Source: CAD feature listing. Evaluate the final solid. Frame: model axes, mm. A direction names the side the tool comes from. Round coordinates to 2 decimals unless told otherwise and drop trailing zeros. Order: outer loops, then holes, each group sorted by start corner. A loop starts at its lowest first (then second) coordinate and runs counter-clockwise, first axis right, second up. Notation, with made-up numbers: M 5.5,22 L 42.5,22 A29 cw 42.5,52 Z; hole C 66.5,-1.5 d8. An arc over 180 degrees is marked long. Answer in a Markdown table with one row per item. Add a question column.
```python
from build123d import *

# Parameters (mm, degrees)
F1_DEPTH = 2.0574
F2_R     = 2.54


with BuildPart() as f1:
    # F0 (on Top) → F1 (new body)
    with BuildSketch(Plane.XY):
        Polygon((-19.05, -6.831449), (0, -7.122084), (0, -4.836785), (-19.05, -4.546149), (-19.05, 5.615033), (-21.59, 5.653784), (-21.59, -16.95388), (-19.05, -16.992631), align=None)
        with BuildLine():
            Line((0, -7.122084), (3.032153, -7.168344))
            ThreePointArc((3.032153, -7.168344), (7.041994, 3.104817), (-2.545553, -2.344551))
            Line((-2.545553, -2.344551), (-0.515844, -2.007228))
            ThreePointArc((-0.515844, -2.007228), (5.158216, 1.472099), (3.187775, -4.885419))
            Line((3.187775, -4.885419), (0, -4.836785))
            Line((0, -4.836785), (0, -7.122084))
        make_face()
    extrude(amount=F1_DEPTH)

    # F2
    f2_edges = [f1.edges().sort_by_distance(p)[0] for p in [
        (-19.05, -6.831449, 1.0287),
        (-19.05, -4.546149, 1.0287),
    ]]
    fillet(f2_edges, radius=F2_R)


solid = f1.part
```
(1) Cut plane A-A (z = 0.6). Return loops of the section in (x, y), and give its area (3 significant figures).
(2) Cut plane B-B (y = -0.25). Return loops of the section in (x, z).
(3) Line query: line 1 (X direction, y = -0.75, z = 1.6); line 2 (X direction, y = 1.25, z = 1.55); line 3 (Y direction, x = 1, z = 0.95). Output: solid intervals per line, ascending. Write a range as from..to.
(4) Access query for faces 1 (the face through (-18.27, -7.58, 1.04)), 2 (the face through (7.19, 2.97, 1.01)), 3 (the face through (-18.3, -3.847, 1.043)). Directions: +Z, -Z, +X, -X, +Y, -Y. A direction counts if a zero-diameter tool reaches every point of the face in a straight line with its end or side. Return the directions, or none.
(5) Cut plane D-D (y = 2.75). Return loops of the section in (x, z).
(6) Pin query (flat end, axial travel): pin 1 (1 mm diameter, centred on y = -9.5, z = 0.5, fed in from +X); pin 2 (1.5 mm diameter, centred on x = -14.5, y = -4.5, fed in from -Z); pin 3 (0.6 mm diameter, centred on y = -13, z = 1.5, fed in from +X). Return the tip coordinate at first contact, or that it passes through.
(7) Cut plane C-C (x = 2.5). Return loops of the section in (y, z).
(8) Draft query along X for faces 4 (the face through (-19.05, -13, 1)), 5 (the face through (-9, -5, 2.057)), 6 (the face through (-1.545, -2.178, 1.014)). Return one class per face: +X half, -X half, draft (parallel to the pull), parting line (faces both ways), or undercut.
Answer list:
| question | item | result |
|---|---|---|
| 1 | outline | M -21.59,-16.95 L -19.05,-16.99 L -19.05,-9.41 A2.54 cw -16.47,-6.87 L 3.03,-7.17 A5.85 ccw long -2.55,-2.34 L -0.52,-2.01 A3.56 cw long 3.19,-4.89 L -16.55,-4.58 A2.54 cw -19.05,-2.04 L -19.05,5.62 L -21.59,5.65 Z |
| 1 | area | 165 mm² |
| 2 | outline | M -21.59,0 L -19.05,0 L -19.05,2.06 L -21.59,2.06 Z; M -2.54,0 L -0.41,0 L -0.41,2.06 L -2.54,2.06 Z; M 6.36,0 L 8.97,0 L 8.97,2.06 L 6.36,2.06 Z |
| 3 | line 1 | -21.59..-19.05, -2.61..-0.53, 6.48..9.04 |
| 3 | line 2 | -21.59..-19.05, -2.04..0.54, 5.42..8.47 |
| 3 | line 3 | -7.14..-4.85, 1.62..4.09 |
| 4 | face 1 | +Z, -Z, -Y |
| 4 | face 2 | +Z, -Z |
| 4 | face 3 | +Z, -Z, +Y |
| 5 | outline | M -21.59,0 L -19.05,0 L -19.05,2.06 L -21.59,2.06 Z; M -0.99,0 L 7.42,0 L 7.42,2.06 L -0.99,2.06 Z |
| 6 | pin 1 | x = -19.02 |
| 6 | pin 2 | z = 0 |
| 6 | pin 3 | x = -19.05 |
| 7 | outline | M -7.16,0 L -4.87,0 L -4.87,2.06 L -7.16,2.06 Z; M 2.19,0 L 4.49,0 L 4.49,2.06 L 2.19,2.06 Z |
| 8 | face 4 | +X half |
| 8 | face 5 | draft |
| 8 | face 6 | undercut |
